from build123d import *

# Parameters (mm, degrees)
EXTRUDE_1_DEPTH      = 10
EXTRUDE_START        = -100
EXTRUDE_3_DEPTH      = 80
SKETCH_5_W           = 80
SKETCH_5_H           = 60
CUT_EXTRUDE_2_DEPTH  = 110
FILLET_1_R           = 50
FILLET_2_R           = 200
SKETCH_16_R          = 13
CUT_EXTRUDE_10_DEPTH = 0.75
CUT_EXTRUDE_START    = -0.75
SKETCH_17_R          = 13
CUT_EXTRUDE_11_DEPTH = 0.75
SKETCH_18_R          = 2.5
EXTRUDE_6_DEPTH      = 200
SKETCH_20_W          = 45.086358536
SKETCH_20_H          = 37.636191029
SKETCH_20_W_2        = 32.7550468
SKETCH_20_H_2        = 44.701005045
CUT_EXTRUDE_12_DEPTH = 322.869538789


with BuildPart() as part:
    # 草图1 → 凸台-拉伸1 (new body)
    with BuildSketch(Plane(origin=(0, 0, 0), x_dir=(1, 0, 0), z_dir=(0, 1, 0))):
        Polygon((-100, 0), (100, 0), (100, 180), (50, 300), (-50, 300), (-100, 180), align=None)
    extrude(amount=EXTRUDE_1_DEPTH)

    # 草图4 → 凸台-拉伸3 (add)
    with BuildSketch(Plane.XY.offset(EXTRUDE_START)):
        with BuildLine():
            Line((0, 29), (0, 10))
            Line((0, 10), (30, 10))
            Line((30, 10), (30, 40))
            ThreePointArc((30, 40), (21.213203436, 61.213203436), (0, 70))
            Line((0, 70), (0, 51))
            ThreePointArc((0, 51), (7.778174593, 47.778174593), (11, 40))
            ThreePointArc((11, 40), (7.778174593, 32.221825407), (0, 29))
        make_face()
        with BuildLine():
            Line((-30, 10), (0, 10))
            Line((0, 10), (0, 29))
            ThreePointArc((0, 29), (-11, 40), (0, 51))
            Line((0, 51), (0, 70))
            ThreePointArc((0, 70), (-21.213203436, 61.213203436), (-30, 40))
            Line((-30, 40), (-30, 10))
        make_face()
    extrude(amount=-EXTRUDE_3_DEPTH)

    # 草图5 → 切除-拉伸2 (cut)
    with BuildSketch(Plane(origin=(0, 10, 0), x_dir=(1, 0, 0), z_dir=(0, 1, 0))):
        with Locations((0, 140)):
            Rectangle(SKETCH_5_W, SKETCH_5_H)
    extrude(amount=CUT_EXTRUDE_2_DEPTH, mode=Mode.SUBTRACT)

    # 圆角1
    fillet_1_edges = [part.edges().sort_by_distance(p)[0] for p in [
        (-50, 5, -300),
        (50, 5, -300),
    ]]
    fillet(fillet_1_edges, radius=FILLET_1_R)

    # 圆角2
    fillet_2_edges = [part.edges().sort_by_distance(p)[0] for p in [
        (-100, 5, -180),
        (100, 5, -180),
    ]]
    fillet(fillet_2_edges, radius=FILLET_2_R)

    # 草图16 → 切除-拉伸10 (cut)
    with BuildSketch(Plane.XY.offset(-100)):
        with Locations((0, 40)):
            Circle(SKETCH_16_R)
    extrude(amount=-CUT_EXTRUDE_10_DEPTH, mode=Mode.SUBTRACT)

    # 草图17 → 切除-拉伸11 (cut)
    with BuildSketch(Plane(origin=(0, 0, -180), x_dir=(-1, 0, 0), z_dir=(0, 0, -1)).offset(CUT_EXTRUDE_START)):
        with Locations(Location((0, 40, 0), (0, 0, 180))):
            Circle(SKETCH_17_R)
    extrude(amount=CUT_EXTRUDE_11_DEPTH, mode=Mode.SUBTRACT)

    # 草图18 → 凸台-拉伸6 (add)
    with BuildSketch(Plane.ZY.offset(100)):
        with BuildLine():
            Line((-40, 10), (-40, 30))
            ThreePointArc((-40, 30), (-30, 40), (-20, 30))
            Line((-20, 30), (-20, 10))
            Line((-20, 10), (-40, 10))
        make_face()
        with Locations((-30, 30)):
            Circle(SKETCH_18_R, mode=Mode.SUBTRACT)
    extrude(amount=-EXTRUDE_6_DEPTH)

    # 草图20 → 切除-拉伸12 (cut, through all)
    with BuildSketch(Plane(origin=(0, 10, 0), x_dir=(1, 0, 0), z_dir=(0, 1, 0))):
        with Locations((-37.543179268, 30.422188826)):
            Rectangle(SKETCH_20_W, SKETCH_20_H)
        with Locations((91.463881936, 29.458805096)):
            Rectangle(SKETCH_20_W_2, SKETCH_20_H_2)
        with Locations((37.543179268, 30.422188826)):
            Rectangle(SKETCH_20_W, SKETCH_20_H)
        with Locations((-91.463881936, 29.458805096)):
            Rectangle(SKETCH_20_W_2, SKETCH_20_H_2)
    extrude(amount=CUT_EXTRUDE_12_DEPTH, mode=Mode.SUBTRACT)


solid = part.part
Verification items for the finished model (mm, model axes). A direction names the side the tool comes from. Coordinates: 2 decimals unless noted, no trailing zeros. Order: outer loops, then holes, each group sorted by start corner. A loop starts at its lowest first (then second) coordinate and runs counter-clockwise, first axis right, second up. Notation, with made-up numbers: (28, 14) -> (53, 14) arc R13 ccw to (53, 31) -> close; hole circle Ø11 at (24, 58). An arc over 180 degrees is marked (long way). Use CSV: the item, a comma, the result in double quotes. Start each with the question number.
Q1. Section check A-A, the plane y = 24. Record the cut outline in (x, z).
Q2. Section check C-C, the plane z = -54. Record the cut outline in (x, y).
Q3. Thickness scan on line 1 along Z through (x, y) = (0.5, 15); line 2 along X through (y, z) = (11.5, -37); line 3 along Z through (x, y) = (-22.5, 40.5). Record the ranges inside material, lowest first.
Q4. Section check B-B, the plane y = 58.5. Record the cut outline in (x, z).
Q5. Section check D-D, the plane x = -49.5. Record the cut outline in (y, z).
Q6. Tool access check on faces 1 (the flat face through (67, 20, -40)), 2 (the flat face through (-30, 25, -105)), 3 (the flat face through (-11, 37, -179.25)), 4 (the flat face through (-68, 20, -20)). Record the directions out of +Z, -Z, +X, -X, +Y, -Y that give a thin tool (end or side, any length) a straight path to the whole face; none if there is none.
Q7. Draft check along X on faces 5 (the flat face through (30, 25, -175)), 6 (the cylindrical face through (-1.69, 27.11, -179.62)), 7 (the flat face through (15, 25, -30)), 8 (the flat face through (-75.086, 25, -30)). Enter one of: +X half, -X half, draft (parallel to the pull), parting line (faces both ways), or undercut.
Q8. Depth check by flat-ended pin: P1, Ø10, axis at y = 28, z = -27.5, coming from the +X side; P2, Ø6, axis at y = 29, z = -28, coming from the -X side; P3, Ø22, axis at x = 5.5, y = 16.5, coming from the +Z side; P4, Ø5, axis at y = 26, z = -173.5, coming from the -X side. Enter the tip coordinate at first touch or a pass-through.
Returned:
1,outline,"(-75.09, -40) -> (-60.09, -40) -> (-60.09, -20) -> (-75.09, -20) -> close; (-30, -180) -> (30, -180) -> (30, -170) -> (-30, -170) -> close; (-30, -110) -> (30, -110) -> (30, -100) -> (-30, -100) -> close; (-15, -40) -> (15, -40) -> (15, -20) -> (-15, -20) -> close; (60.09, -40) -> (75.09, -40) -> (75.09, -20) -> (60.09, -20) -> close"
2,outline,"(-100, 0) -> (100, 0) -> (100, 10) -> (-100, 10) -> close"
3,line 1,"z = -180 to -170, -110 to -100, -40 to -20"
3,line 2,"x = -75.09 to -60.09, -15 to 15, 60.09 to 75.09"
3,line 3,"z = -180 to -170, -110 to -100"
4,outline,"(-23.62, -180) -> (23.62, -180) -> (23.62, -170) -> (-23.62, -170) -> close; (-23.62, -110) -> (23.62, -110) -> (23.62, -100) -> (-23.62, -100) -> close"
5,outline,"(0, -287.71) -> (10, -287.71) -> (10, 0) -> (0, 0) -> close"
6,face 1,"-Z, +X, -X, +Y"
6,face 2,"+Z, -Z, -X, +Y"
6,face 3,"-Z"
6,face 4,"+Z, +X, -X, +Y"
7,face 5,"+X half"
7,face 6,"undercut"
7,face 7,"undercut"
7,face 8,"-X half"
8,P1,"stops at x = 75.09"
8,P2,"stops at x = -75.09"
8,P3,"stops at z = 0"
8,P4,"stops at x = -30"
